Source: three-view drawing plus pictorial views. Frame: mm from the lowest corner of the part. A direction names the side the tool comes from. Coordinates: 2 decimals unless noted, no trailing zeros. Loops run counter-clockwise (first coordinate to the right, second up) from the corner with the lowest first, then second, coordinate; pieces in that order, holes last. Notation, with made-up numbers: (0.25, 56.25) - (33.25, 56.25) arc R9 ccw to (33.25, 64.25) - close; hole circle Ø4 at (15, -17.75). An arc over 180 degrees is marked (long way). Return JSON: item names as keys, results as strings.
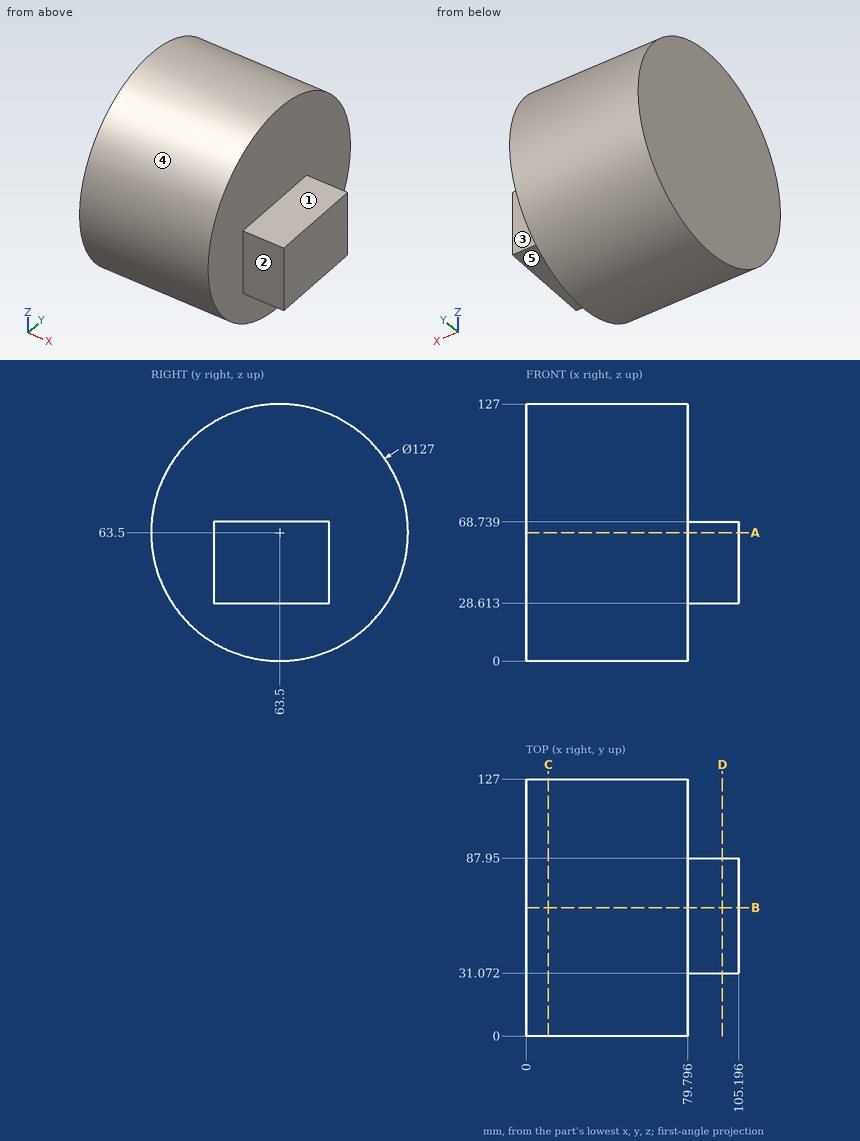
Item 1: First-contact query: pin 1 Ø12 at (x, z) = (48.5, 95) entering from -Y (1 decimal); pin 2 Ø6 at (x, z) = (44, 86) entering from -Y; pin 3 Ø7.5 at (x, y) = (98, 73) entering from +Z. Flat tips, straight axial feed; report the tip coordinate or a pass-through.
Worked out:
{"pin 1": "y = 5.3", "pin 2": "y = 3.07", "pin 3": "z = 68.74"}
Item 2: Section query B-B, the plane y = 63.5. Return loops of the section in (x, z), and give its area (3 significant figures).
Worked out:
{"outline": "(0, 0) - (79.8, 0) - (79.8, 28.61) - (105.2, 28.61) - (105.2, 68.74) - (79.8, 68.74) - (79.8, 127) - (0, 127) - close", "area": "11,200 mm^2"}
Item 3: Ray query, probe 1 along X at (y, z) = (96.5, 21); probe 2 along Z at (x, y) = (98, 84.5); probe 3 along Y at (x, z) = (85.5, 61). Return the intervals inside material, ascending. Write a range as from..to.
Worked out:
{"probe 1": "0..79.8", "probe 2": "28.61..68.74", "probe 3": "31.07..87.95"}
Item 4: Section query D-D, the plane x = 97. Return loops of the section in (y, z).
Worked out:
{"outline": "(31.07, 28.61) - (87.95, 28.61) - (87.95, 68.74) - (31.07, 68.74) - close"}
Item 5: Reachability of the marked faces 1, 2, 3, 4 and 5 from +Z, -Z, +X, -X, +Y, -Y: full face, straight path, thin tool, end or side. Return the list, or none.
Worked out:
{"face 1": "+Z, +X, +Y, -Y", "face 2": "+Z, -Z, +X, -Y", "face 3": "+Z, -Z, +X, +Y", "face 4": "+X, -X", "face 5": "-Z, +X, +Y, -Y"}
Item 6: Section query A-A, the plane z = 63.5. Return loops of the section in (x, y), and give its area (3 significant figures).
Worked out:
{"outline": "(0, 0) - (79.8, 0) - (79.8, 31.07) - (105.2, 31.07) - (105.2, 87.95) - (79.8, 87.95) - (79.8, 127) - (0, 127) - close", "area": "11,600 mm^2"}
Item 7: Section query C-C, the plane x = 11. Return loops of the section in (y, z), and give its area (3 significant figures).
Worked out:
{"outline": "circle Ø127 at (63.5, 63.5)", "area": "12,700 mm^2"}
